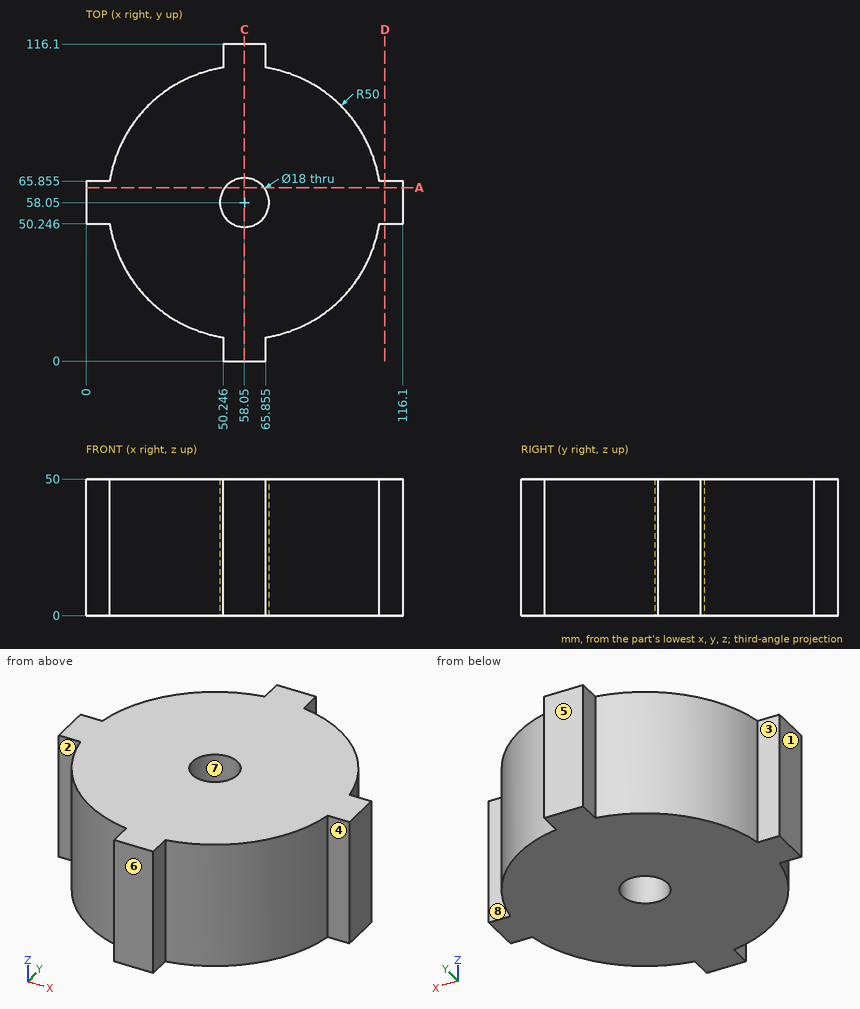
Drawing for the job (mm, zero at the part's lowest x, y, z). A direction names the side the tool comes from. Round coordinates to 2 decimals unless told otherwise and drop trailing zeros. Order: outer loops, then holes, each group sorted by start corner. A loop starts at its lowest first (then second) coordinate and runs counter-clockwise, first axis right, second up. Notation, with made-up numbers: (-30, 8) -> (-24, 8) arc R22 cw to (-24, 41) -> close; hole circle Ø5 at (42.25, -22.75). An arc over 180 degrees is marked (long way). Write item = value, one per line. Start each with the question number.
(1) Pull direction Y, two halves, no side cores. Call the marked faces 6, 7 and 8: released by +Y, released by -Y, zero draft, split by the parting line, or undercut.
(2) Cut at C-C, the plane x = 58. List the corners of the cut face in (y, z), then the cut area to 4 significant figures.
(3) Pin check, flat tips, straight feed: P1, Ø4.5, axis at y = 4, z = 30.5, coming from the -X side; P2, Ø7, axis at y = 5, z = 30, coming from the +X side (1 decimal); P3, Ø1, axis at y = 38.5, z = 19.5, coming from the -X side. Stop position of each tip, or through.
(4) Cut at D-D, the plane x = 109.5. List the corners of the cut face in (y, z) (1 decimal).
(5) Cut at A-A, the plane y = 63.5. List the corners of the cut face in (x, z).
(6) Which spindle directions (+Z, -Z, +X, -X, +Y, -Y) get a long thin tool onto all of the face, cutting with end or side? Do the marked faces 1, 2, 3, 4 and 5. Say none if no direction does.
(7) Probe line 1 (Y direction, x = 62.5, z = 12); line 2 (X direction, y = 58.5, z = 7.5); line 3 (Y direction, x = 51.5, z = 48.5). List the from-to ranges inside material, lowest first. Write a range as [from, to].
Model answer:
q1.face_6 = released by -Y
q1.face_7 = undercut
q1.face_8 = released by +Y
q2.outline = (0, 0) -> (49.05, 0) -> (49.05, 50) -> (0, 50) -> close; (67.05, 0) -> (116.1, 0) -> (116.1, 50) -> (67.05, 50) -> close
q2.area = 4,905 mm2
q3.P1 = 50.25
q3.P2 = 65.9
q3.P3 = 11.82
q4.outline = (50.2, 0) -> (65.9, 0) -> (65.9, 50) -> (50.2, 50) -> close
q5.outline = (0, 0) -> (50.89, 0) -> (50.89, 50) -> (0, 50) -> close; (65.21, 0) -> (116.1, 0) -> (116.1, 50) -> (65.21, 50) -> close
q6.face_1 = +Z, -Z, -X, +Y, -Y
q6.face_2 = +Z, -Z, -X, -Y
q6.face_3 = +Z, -Z, -X, +Y
q6.face_4 = +Z, -Z, +X, -Y
q6.face_5 = +Z, -Z, +X, -X, +Y
q7.line_1 = [0, 50.23], [65.87, 116.1]
q7.line_2 = [0, 49.06], [67.04, 116.1]
q7.line_3 = [0, 51.88], [64.22, 116.1]
